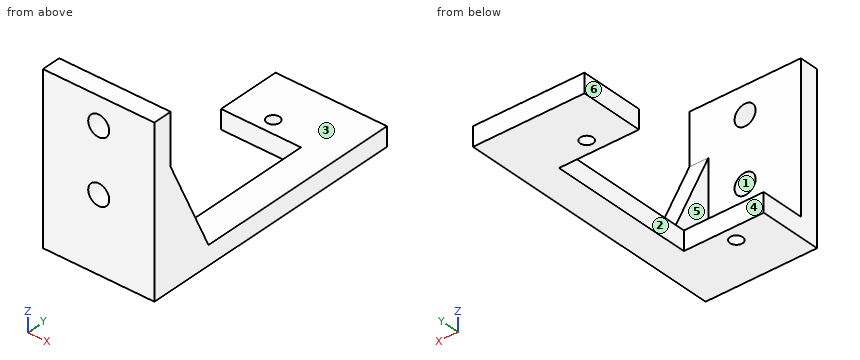
from build123d import *

# Parameters (mm, degrees)
SKETCH_1_W          = 17.5
SKETCH_1_H          = 23
SKETCH_1_R          = 1.65
EXTRUDE_1_DEPTH     = 3
SKETCH_2_W          = 17.5
SKETCH_2_H          = 3
EXTRUDE_2_DEPTH     = 43
SKETCH_3_R          = 1
SKETCH_3_W          = 12.55
SKETCH_3_H          = 23.07
CUT_EXTRUDE_1_DEPTH = 3
EXTRUDE_3_DEPTH     = 3


with BuildPart() as part:
    # 草图1 → 凸台-拉伸1 (new body)
    with BuildSketch(Plane(origin=(0, 0, 0), x_dir=(1, 0, 0), z_dir=(0, 1, 0))):
        Rectangle(SKETCH_1_W, SKETCH_1_H)
        with Locations(Location((0, 2.85, 0), (0, 0, 270))):
            Circle(SKETCH_1_R, mode=Mode.SUBTRACT)
        with Locations(Location((0, -7.15, 0), (0, 0, 270))):
            Circle(SKETCH_1_R, mode=Mode.SUBTRACT)
    extrude(amount=EXTRUDE_1_DEPTH)

    # 草图2 → 凸台-拉伸2 (add)
    with BuildSketch(Plane(origin=(0, 0, 0), x_dir=(1, 0, 0), z_dir=(0, 1, 0))):
        with Locations((0, 13)):
            Rectangle(SKETCH_2_W, SKETCH_2_H)
    extrude(amount=EXTRUDE_2_DEPTH)

    # 草图3 → 切除-拉伸1 (cut)
    with BuildSketch(Plane(origin=(0, 0, -14.5), x_dir=(-1, 0, 0), z_dir=(0, 0, -1))):
        with Locations((2.5, 7.55)):
            Circle(SKETCH_3_R)
        with Locations((2.5, 35.22)):
            Circle(SKETCH_3_R)
        with Locations((2.475, 21.385)):
            Rectangle(SKETCH_3_W, SKETCH_3_H)
    extrude(amount=-CUT_EXTRUDE_1_DEPTH, mode=Mode.SUBTRACT)

    # 草图4 → 凸台-拉伸3 (add)
    with BuildSketch(Plane(origin=(8.75, 0, 0), x_dir=(0, 0, -1), z_dir=(1, 0, 0))):
        Polygon((11.5, 3), (-3.5, 3), (11.5, 10), align=None)
    extrude(amount=-EXTRUDE_3_DEPTH)


solid = part.part
Read the model definition and answer for the solid it produces. Units are mm, in the model's axes. Face numbers are marked on the shaded views. A direction names the side the tool comes from. Round coordinates to 2 decimals unless told otherwise and drop trailing zeros. Loops run counter-clockwise (first coordinate to the right, second up) from the corner with the lowest first, then second, coordinate; pieces in that order, holes last.
Q1. Section C-C on z = 6 is taken. Write down the section's boundary in (x, y), and give its area (3 significant figures).
Q2. Section A-A on y = 35.22 is taken. Write down the section's boundary in (x, z).
Q3. Which of the six approach directions +Z, -Z, +X, -X, +Y, -Y give full straight-line access (tool end or side, diameter ignored) to the marked faces 4, 5 and 6?
Q4. Determine the mould class of the marked faces 1, 2 and 3 for opening direction Z: released by +Z, released by -Z, zero draft, split by the parting line, or undercut.
Q5. Each of these flat-tipped pins is pushed along its axis until it touches: pin 1 (2.5 mm diameter, centred on y = 21, z = -13.5, fed in from -X); pin 2 (3 mm diameter, centred on x = 0, z = 7.15, fed in from -Y); pin 3 (2.5 mm diameter, centred on x = -2.5, y = 35.22, fed in from +Z); pin 4 (8 mm diameter, centred on x = -4.5, z = 0.5, fed in from +Y). Where does it stop, or does it pass through?
Q6. Consider probe 1 along Y at (x, z) = (-2.5, -12.6); probe 2 along X at (y, z) = (2.15, -2.85); probe 3 along Y at (x, z) = (-3, -6.75). Determine where each line is inside the solid, lowest interval first.
Q7. Section D-D on x = -4.25 is taken. Write down the section's boundary in (y, z), and give its area (3 significant figures).
Q8. Section B-B on x = 0 is taken. Write down the section's boundary in (y, z), and give its area (3 significant figures).
Output:
1. outline: (-8.75, 0) - (-1.18, 0) - (-1.18, 3) - (-8.75, 3) - close; (1.18, 0) - (8.75, 0) - (8.75, 3) - (1.18, 3) - close
1. area: 45.4 mm2
2. outline: (-8.75, -14.5) - (-3.5, -14.5) - (-3.5, -11.5) - (-8.75, -11.5) - close; (-1.5, -14.5) - (8.75, -14.5) - (8.75, -11.5) - (-1.5, -11.5) - close
3. face 4: +Z, -Z, -X
3. face 5: +Z, -X, +Y
3. face 6: +Z, -Z, -X, +Y, -Y
4. face 1: undercut
4. face 2: zero draft
4. face 3: released by +Z
5. pin 1: stops at x = 3.8
5. pin 2: passes through
5. pin 3: stops at z = -11.5
5. pin 4: stops at y = 3
6. probe 1: y = 0 to 6.55, 8.55 to 9.85, 32.92 to 34.22, 36.22 to 43
6. probe 2: x = -8.75 to -1.65, 1.65 to 8.75
6. probe 3: y = 0 to 3
7. outline: (0, -14.5) - (9.85, -14.5) - (9.85, -11.5) - (3, -11.5) - (3, 11.5) - (0, 11.5) - close; (32.92, -14.5) - (43, -14.5) - (43, -11.5) - (32.92, -11.5) - close
7. area: 129 mm2
8. outline: (0, -14.5) - (9.85, -14.5) - (9.85, -11.5) - (3, -11.5) - (3, -4.5) - (0, -4.5) - close; (0, -1.2) - (3, -1.2) - (3, 5.5) - (0, 5.5) - close; (0, 8.8) - (3, 8.8) - (3, 11.5) - (0, 11.5) - close; (32.92, -14.5) - (43, -14.5) - (43, -11.5) - (32.92, -11.5) - close
8. area: 109 mm2
